from build123d import *

# Parameters (mm, degrees)
EXTRUDE_1_DEPTH     = 3
EXTRUDE_1_2_DEPTH   = 3
SKETCH_2_W          = 17.5
SKETCH_2_H          = 3
SKETCH_2_W_2        = 3
SKETCH_2_H_2        = 20
EXTRUDE_2_DEPTH     = 43
SKETCH_3_W          = 55
SKETCH_3_H          = 3
EXTRUDE_3_DEPTH     = 10
EXTRUDE_4_DEPTH     = 2.5
SKETCH_5_R          = 3
CUT_EXTRUDE_1_DEPTH = 2.6
SKETCH_7_R          = 1.625
CUT_EXTRUDE_2_DEPTH = 118.972920622
SKETCH_8_W          = 5.5
SKETCH_8_H          = 30
EXTRUDE_5_DEPTH     = 5


with BuildPart() as part:
    # Sketch 1 → Extrude 1 (new body)
    with BuildSketch(Plane(origin=(0, 0, 0), x_dir=(1, 0, 0), z_dir=(0, 1, 0))):
        Polygon((27.5, 25.5), (45, 25.5), (45, 10), (53, 10), (53, -10), (45, -10), (45, -25.5), (27.5, -25.5), align=None)
    extrude(amount=EXTRUDE_1_DEPTH)



with BuildPart() as body_2:
    # Sketch 1 → Extrude 1 2 (new body)
    with BuildSketch(Plane(origin=(0, 0, 0), x_dir=(1, 0, 0), z_dir=(0, 1, 0))):
        Polygon((-27.5, -25.5), (-27.5, 25.5), (-45, 25.5), (-45, 10), (-53, 10), (-53, -10), (-45, -10), (-45, -25.5), align=None)
    extrude(amount=EXTRUDE_1_2_DEPTH)


with BuildPart() as part_1:
    add(part.part)

    add(body_2.part)  # Extrude 2 merges body 2
    # Sketch 2 → Extrude 2 (add)
    with BuildSketch(Plane(origin=(0, 3, 0), x_dir=(1, 0, 0), z_dir=(0, 1, 0))):
        with Locations((36.25, 24)):
            Rectangle(SKETCH_2_W, SKETCH_2_H)
        with Locations((51.5, 0)):
            Rectangle(SKETCH_2_W_2, SKETCH_2_H_2)
        with Locations((36.25, -24)):
            Rectangle(SKETCH_2_W, SKETCH_2_H)
        with Locations((-36.25, -24)):
            Rectangle(SKETCH_2_W, SKETCH_2_H)
        with Locations((-51.5, 0)):
            Rectangle(SKETCH_2_W_2, SKETCH_2_H_2)
        with Locations((-36.25, 24)):
            Rectangle(SKETCH_2_W, SKETCH_2_H)
    extrude(amount=EXTRUDE_2_DEPTH)

    # Sketch 3 → Extrude 3 (add)
    with BuildSketch(Plane(origin=(0, 46, 0), x_dir=(1, 0, 0), z_dir=(0, 1, 0))):
        Polygon((45, 25.5), (53, 25.5), (53, 10), (50, 10), (50, 22.5), (45, 22.5), align=None)
        with Locations((0, 24)):
            Rectangle(SKETCH_3_W, SKETCH_3_H)
        Polygon((-45, 22.5), (-45, 25.5), (-53, 25.5), (-53, 10), (-50, 10), (-50, 22.5), align=None)
        Polygon((-45, -25.5), (-53, -25.5), (-53, -10), (-50, -10), (-50, -22.5), (-45, -22.5), align=None)
        Polygon((45, -22.5), (45, -25.5), (53, -25.5), (53, -10), (50, -10), (50, -22.5), align=None)
        with Locations((0, -24)):
            Rectangle(SKETCH_3_W, SKETCH_3_H)
    extrude(amount=-EXTRUDE_3_DEPTH)

    # Sketch 4 → Extrude 4 (add)
    with BuildSketch(Plane.ZY.offset(53)):
        Polygon((-10, 26), (10, 26), (10, 36), (15, 36), (15, 46), (-15, 46), (-15, 36), (-10, 36), align=None)
    extrude_4 = extrude(amount=EXTRUDE_4_DEPTH)

    # Sketch 5 → Cut-Extrude 1 (cut)
    with BuildSketch(Plane(origin=(-50, 0, 0), x_dir=(0, 0, -1), z_dir=(1, 0, 0))):
        with Locations((-6, 41)):
            Circle(SKETCH_5_R)
        with Locations((0, 32)):
            Circle(SKETCH_5_R)
        with Locations(Location((6, 41, 0), (0, 0, 180))):
            Circle(SKETCH_5_R)
    cut_extrude_1 = extrude(amount=-CUT_EXTRUDE_1_DEPTH, mode=Mode.SUBTRACT)

    # Sketch 7 → Cut-Extrude 2 (cut, through all)
    with BuildSketch(Plane(origin=(-52.6, 0, 0), x_dir=(0, 0, -1), z_dir=(1, 0, 0))):
        with Locations((-6, 41)):
            Circle(SKETCH_7_R)
        with Locations((6, 41)):
            Circle(SKETCH_7_R)
        with Locations((0, 32)):
            Circle(SKETCH_7_R)
    cut_extrude_2 = extrude(amount=-CUT_EXTRUDE_2_DEPTH, mode=Mode.SUBTRACT)

    # Mirror 2: Extrude 4, Cut-Extrude 1, Cut-Extrude 2 across plane
    add(extrude_4.mirror(Plane(origin=(0, 0, 0), x_dir=(0, 0, 1), z_dir=(1, 0, 0))))
    add(cut_extrude_1.mirror(Plane(origin=(0, 0, 0), x_dir=(0, 0, 1), z_dir=(1, 0, 0))), mode=Mode.SUBTRACT)
    add(cut_extrude_2.mirror(Plane(origin=(0, 0, 0), x_dir=(0, 0, 1), z_dir=(1, 0, 0))), mode=Mode.SUBTRACT)

    # Sketch 8 → Extrude 5 (add)
    with BuildSketch(Plane(origin=(0, 46, 0), x_dir=(1, 0, 0), z_dir=(0, 1, 0))):
        with Locations((-52.75, 0)):
            Rectangle(SKETCH_8_W, SKETCH_8_H)
        with Locations((52.75, 0)):
            Rectangle(SKETCH_8_W, SKETCH_8_H)
    extrude(amount=EXTRUDE_5_DEPTH)


solid = part_1.part
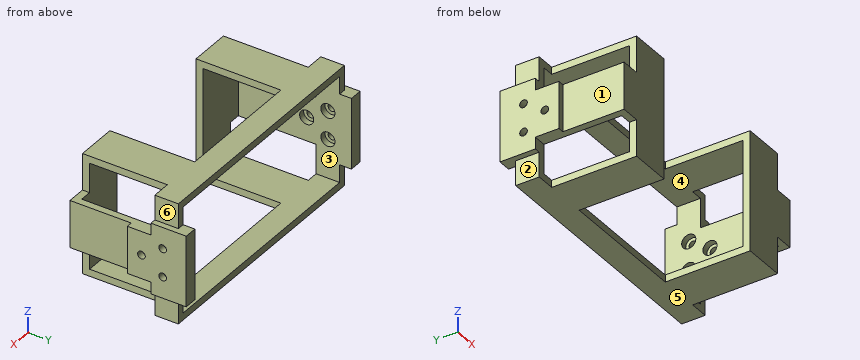
Here's how the part is built. I have some questions about the finished solid (model axes, mm). Face numbers are marked on the shaded views. A direction names the side the tool comes from. Give positions to 0.01 mm unless a question says otherwise; leave off trailing zeros. Loops run counter-clockwise (first coordinate to the right, second up) from the corner with the lowest first, then second, coordinate; pieces in that order, holes last. Notation, with made-up numbers: (-13.75, 82.5) -> (43.25, 82.5) arc R22 cw to (43.25, 97.5) -> close; hole circle Ø9 at (23.5, 37). An arc over 180 degrees is marked (long way). One line per item, written item: value.
Q1. Suppose I cut it at D-D on z = -18.5. Please give me the cut outline in (x, y), then the cut area to 3 significant figures.
Answers follow:
outline: (-53, 36) -> (-50, 36) -> (-50, 46) -> (-53, 46) -> close; (-45, 0) -> (-27.5, 0) -> (-27.5, 3) -> (-45, 3) -> close; (27.5, 0) -> (45, 0) -> (45, 3) -> (27.5, 3) -> close; (50, 36) -> (53, 36) -> (53, 46) -> (50, 46) -> close
area: 165 mm^2
Q2. Suppose I cut it at C-C on x = 19.5. Please give me the cut outline in (y, z), then the cut area to 3 significant figures.
Answers follow:
outline: (36, -25.5) -> (46, -25.5) -> (46, -22.5) -> (36, -22.5) -> close; (36, 22.5) -> (46, 22.5) -> (46, 25.5) -> (36, 25.5) -> close
area: 60.0 mm^2
Q3. If I drill on line 1 along Z through (x, y) = (34, 17); line 2 along X through (y, z) = (28.5, -3); line 3 along Z through (x, y) = (53.3, 41) (3 decimals), over which ranges is the centre line in solid material (lowest first)?
Answers follow:
line 1: -25.5 to -22.5, 22.5 to 25.5
line 2: -55.5 to -50, 50 to 55.5
line 3: -15 to -7.625, -4.375 to 4.375, 7.625 to 15
Q4. On a 3-axis mill with a long thin cutter (end or side, diameter ignored), from which of +Z, -Z, +X, -X, +Y, -Y can I reach the whole of each face in a straight line? I mean the marked faces 1, 2 and 3. Say none if no direction works.
Answers follow:
face 1: +Z, -Z, -X, -Y
face 2: -Z, -X, +Y, -Y
face 3: +Y
Q5. Suppose I cut it at A-A on z = -6. State how many separate pieces and enclosed holes the cut face has, then the cut area to 3 significant figures.
Answers follow:
separate pieces: 4
enclosed holes: 0
area: 516 mm^2
Q6. We'd pull the mould along X, two halves only. Please class the marked faces 4, 5 and 6: pulls with the +X half, pulls with the -X half, needs draft (parallel to the pull), parting line crosses it, or undercut.
Answers follow:
face 4: undercut
face 5: needs draft
face 6: pulls with the +X half
Q7. I'm going to push flat-ended pins straight in: pin 1 Ø4 at (y, z) = (41, 6) entering from -X; pin 2 Ø2 at (x, z) = (-37.5, 20) entering from +Y; pin 3 Ø11.5 at (x, y) = (-51.5, 17.5) entering from -Z; pin 4 Ø2.5 at (x, z) = (9.5, 24) entering from -Y. Where does each tip first touch, or does it pass through?
Answers follow:
pin 1: x = -55.5
pin 2: y = 3
pin 3: z = -10
pin 4: y = 36
Q8. Suppose I cut it at B-B on y = 18.5. Please give me the cut outline in (x, z).
Answers follow:
outline: (-53, -10) -> (-50, -10) -> (-50, 10) -> (-53, 10) -> close; (-45, -25.5) -> (-27.5, -25.5) -> (-27.5, -22.5) -> (-45, -22.5) -> close; (-45, 22.5) -> (-27.5, 22.5) -> (-27.5, 25.5) -> (-45, 25.5) -> close; (27.5, -25.5) -> (45, -25.5) -> (45, -22.5) -> (27.5, -22.5) -> close; (27.5, 22.5) -> (45, 22.5) -> (45, 25.5) -> (27.5, 25.5) -> close; (50, -10) -> (53, -10) -> (53, 10) -> (50, 10) -> close
